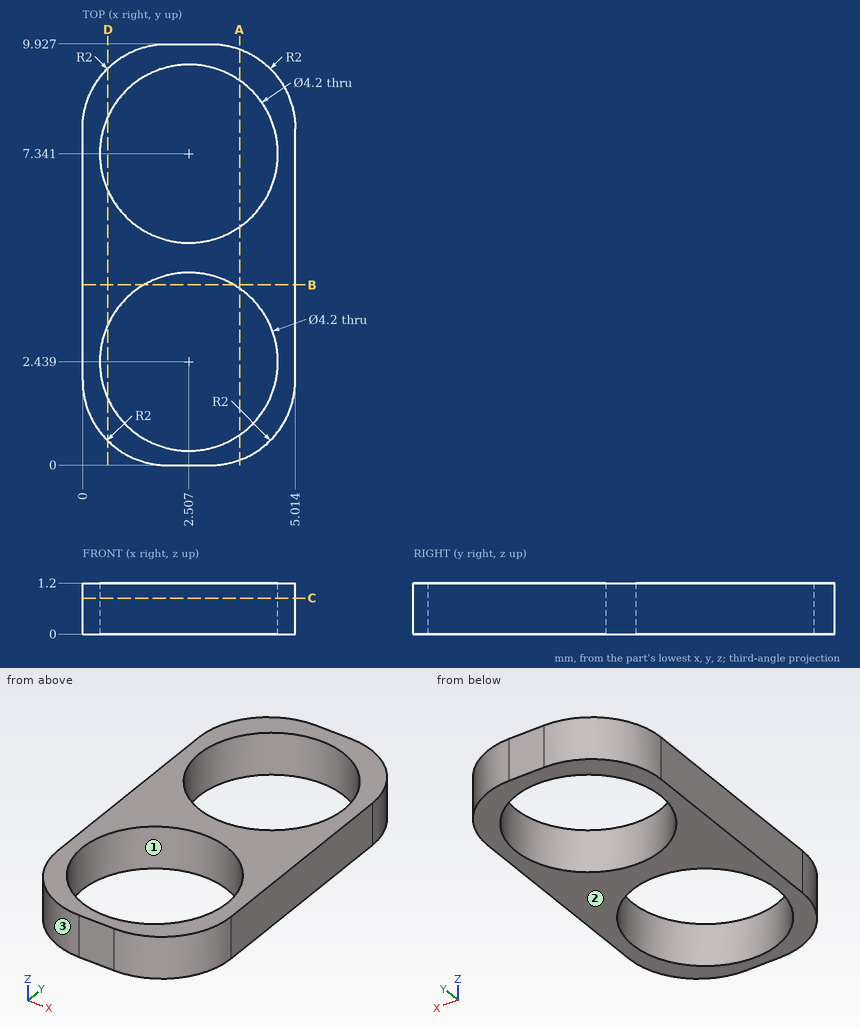
Design review of the part shown in the three views and the two pictorial views. Dimensions are in mm from the part's minimum x, y and z. Give positions to 0.01 mm unless a question says otherwise; leave off trailing zeros. Loops run counter-clockwise (first coordinate to the right, second up) from the corner with the lowest first, then second, coordinate; pieces in that order, holes last. Notation, with made-up numbers: (6, -2) -> (22, -2) arc R11 cw to (22, 18) -> close; hole circle Ø9 at (11.25, 47.25). An arc over 180 degrees is marked (long way). Write each question's results on one line, items separated by ' | '.
Q1. Take a section at A-A, the plane x = 3.7. Write out the cut boundary in (y, z) (1 decimal).
Reply:
outline: (0.1, 0) -> (0.7, 0) -> (0.7, 1.2) -> (0.1, 1.2) -> close; (4.2, 0) -> (5.6, 0) -> (5.6, 1.2) -> (4.2, 1.2) -> close; (9.1, 0) -> (9.8, 0) -> (9.8, 1.2) -> (9.1, 1.2) -> close
Q2. Take a section at D-D, the plane x = 0.6. Write out the cut boundary in (y, z) (1 decimal).
Reply:
outline: (0.6, 0) -> (1.6, 0) -> (1.6, 1.2) -> (0.6, 1.2) -> close; (3.3, 0) -> (6.5, 0) -> (6.5, 1.2) -> (3.3, 1.2) -> close; (8.2, 0) -> (9.4, 0) -> (9.4, 1.2) -> (8.2, 1.2) -> close
Q3. The part is to be moulded in two halves that separate along X. For the marked faces 1, 2 and 3, say which applies: +X half, -X half, draft (parallel to the pull), parting line (faces both ways), or undercut.
Reply:
face 1: undercut | face 2: draft | face 3: -X half
Q4. Take a section at B-B, the plane y = 4.25. Write out the cut boundary in (x, z).
Reply:
outline: (0, 0) -> (1.44, 0) -> (1.44, 1.2) -> (0, 1.2) -> close; (3.57, 0) -> (5.01, 0) -> (5.01, 1.2) -> (3.57, 1.2) -> close
Q5. For pin 1 Ø1 at (x, y) = (4.5, 7) entering from -Z; pin 2 Ø2.5 at (x, y) = (2.51, 2.44) entering from +Z, all flat-tipped, find the tip position at first contact; note any pin that passes through.
Reply:
pin 1: stops at z = 0 | pin 2: passes through
Q6. Wall thickness on L1, parallel to Y at x = 2.5, z = 1.05; L2, parallel to Y at x = 2.75, z = 0.45 (1 decimal); L3, parallel to X at y = 3.75, z = 0.5 (1 decimal): over which ranges is each line inside the solid? List them lowest first.
Reply:
L1: y = 0 to 0.34, 4.54 to 5.24, 9.44 to 9.93 | L2: y = 0 to 0.4, 4.5 to 5.3, 9.4 to 9.9 | L3: x = 0 to 0.9, 4.1 to 5
Q7. Take a section at C-C, the plane z = 0.85. Write out the cut boundary in (x, y).
Reply:
outline: (0, 2) arc R2 ccw to (2, 0) -> (3.01, 0) arc R2 ccw to (5.01, 2) -> (5.01, 7.93) arc R2 ccw to (3.01, 9.93) -> (2, 9.93) arc R2 ccw to (0, 7.93) -> close; hole circle Ø4.2 at (2.51, 2.44); hole circle Ø4.2 at (2.51, 7.34)
